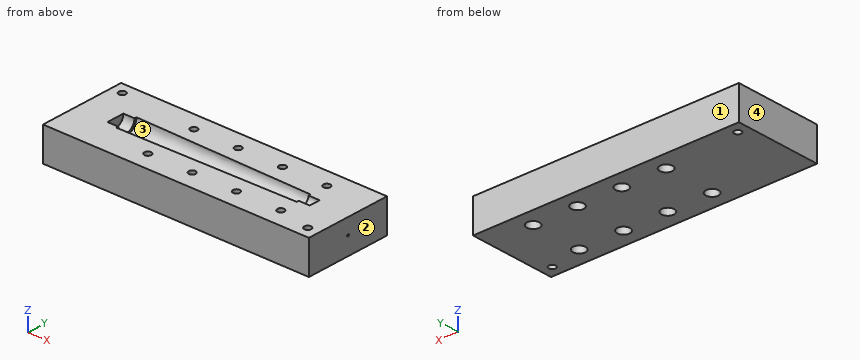
```python
from build123d import *

# Parameters (mm, degrees)
SKIZZE2_W                        = 120
SKIZZE2_H                        = 39.364160046
AUFSATZ_LINEAR_AUSTRAGEN1_DEPTH  = 30
SKIZZE24_R                       = 1.55
SCHNITT_LINEAR_AUSTRAGEN4_DEPTH  = 130.805766806
SKIZZE46_R                       = 2.85
SCHNITT_LINEAR_AUSTRAGEN15_DEPTH = 10
SCHNITT_LINEAR_START             = -5
SCHNITT_LINEAR_AUSTRAGEN25_DEPTH = 2.7
LINEARES_MUSTER1_COUNT           = 4
LINEARES_MUSTER1_PITCH           = 20
SPIEGELN2_COPY_1_SKETCH_R        = 2.85
SPIEGELN2_COPY_1_DEPTH           = 10
SPIEGELN2_COPY_2_SKETCH_R        = 2.85
SPIEGELN2_COPY_2_DEPTH           = 10
SPIEGELN2_COPY_3_SKETCH_R        = 2.85
SPIEGELN2_COPY_3_DEPTH           = 10
SPIEGELN2_START                  = -5
SPIEGELN2_COPY_4_DEPTH           = 2.7
SPIEGELN2_COPY_5_DEPTH           = 2.7
SPIEGELN2_COPY_6_DEPTH           = 2.7
SKIZZE51_R                       = 1.55
SCHNITT_LINEAR_AUSTRAGEN26_DEPTH = 130.805766806
SKIZZE75_R                       = 0.75
SCHNITT_LINEAR_AUSTRAGEN28_DEPTH = 10
SKIZZE76_R                       = 2
SCHNITT_LINEAR_AUSTRAGEN29_DEPTH = 6
SKIZZE80_R                       = 0.5
SCHNITT_LINEAR_AUSTRAGEN34_DEPTH = 21
SCHNITT_LINEAR_START_2           = -7.5
SKIZZE81_R                       = 0.5
SCHNITT_LINEAR_AUSTRAGEN36_DEPTH = 5
ABSPALTEN3_START                 = 15
ABSPALTEN3_OUTLINE_W             = 120
ABSPALTEN3_OUTLINE_H             = 39.364160046
ABSPALTEN3_OUTLINE_R             = 1.55
ABSPALTEN3_DEPTH                 = 15


# Read off the part's stored shape, not the designer's step: Abspalten3
with BuildPart() as part:
    # Skizze2 → Aufsatz-Linear austragen1 (new body)
    with BuildSketch(Plane.XY):
        with Locations((60, 19.682080023)):
            Rectangle(SKIZZE2_W, SKIZZE2_H)
    extrude(amount=AUFSATZ_LINEAR_AUSTRAGEN1_DEPTH)

    # Skizze24 → Schnitt-Linear austragen4 (cut, through all)
    with BuildSketch(Plane.XY.offset(30)):
        with Locations((40, 31.364160046)):
            Circle(SKIZZE24_R)
        with Locations((60, 31.364160046)):
            Circle(SKIZZE24_R)
        with Locations((80, 31.364160046)):
            Circle(SKIZZE24_R)
        with Locations((100, 31.364160046)):
            Circle(SKIZZE24_R)
    schnitt_linear_austragen4 = extrude(amount=-SCHNITT_LINEAR_AUSTRAGEN4_DEPTH, mode=Mode.SUBTRACT)

    # Skizze46 → Schnitt-Linear austragen15 (cut)
    with BuildSketch(Plane(origin=(0, 0, 0), x_dir=(-1, 0, 0), z_dir=(0, 0, -1))):
        with Locations((-100, 31.364160046)):
            Circle(SKIZZE46_R)
    schnitt_linear_austragen15 = extrude(amount=-SCHNITT_LINEAR_AUSTRAGEN15_DEPTH, mode=Mode.SUBTRACT)

    # Skizze50 → Schnitt-Linear austragen25 (cut)
    with BuildSketch(Plane.XY.offset(30).offset(SCHNITT_LINEAR_START)):
        Polygon((97.15, 33.009608314), (97.15, 39.364160046), (102.85, 39.364160046), (102.85, 33.009608314), (102.85, 29.718711779), (100, 28.073263512), (97.15, 29.718711779), align=None)
    schnitt_linear_austragen25 = extrude(amount=-SCHNITT_LINEAR_AUSTRAGEN25_DEPTH, mode=Mode.SUBTRACT)

    # Lineares Muster1: Schnitt-Linear austragen15, Schnitt-Linear austragen25 ×4
    with Locations(*[(-i * LINEARES_MUSTER1_PITCH, 0, 0) for i in range(1, LINEARES_MUSTER1_COUNT)]):
        add(schnitt_linear_austragen15, mode=Mode.SUBTRACT)
        add(schnitt_linear_austragen25, mode=Mode.SUBTRACT)

    # Spiegeln2: Schnitt-Linear austragen15, Schnitt-Linear austragen25 across plane
    add(schnitt_linear_austragen15.mirror(Plane.ZX.offset(19.764160046)), mode=Mode.SUBTRACT)
    add(schnitt_linear_austragen25.mirror(Plane.ZX.offset(19.764160046)), mode=Mode.SUBTRACT)

    # Spiegeln2 copy 1 sketch → Spiegeln2 copy 1 (cut)
    with BuildSketch(Plane(origin=(-20, 39.528320093, 0), x_dir=(-1, 0, 0), z_dir=(0, 0, -1))):
        with Locations((-100, -31.364160046)):
            Circle(SPIEGELN2_COPY_1_SKETCH_R)
    extrude(amount=-SPIEGELN2_COPY_1_DEPTH, mode=Mode.SUBTRACT)

    # Spiegeln2 copy 2 sketch → Spiegeln2 copy 2 (cut)
    with BuildSketch(Plane(origin=(-40, 39.528320093, 0), x_dir=(-1, 0, 0), z_dir=(0, 0, -1))):
        with Locations((-100, -31.364160046)):
            Circle(SPIEGELN2_COPY_2_SKETCH_R)
    extrude(amount=-SPIEGELN2_COPY_2_DEPTH, mode=Mode.SUBTRACT)

    # Spiegeln2 copy 3 sketch → Spiegeln2 copy 3 (cut)
    with BuildSketch(Plane(origin=(-60, 39.528320093, 0), x_dir=(-1, 0, 0), z_dir=(0, 0, -1))):
        with Locations((-100, -31.364160046)):
            Circle(SPIEGELN2_COPY_3_SKETCH_R)
    extrude(amount=-SPIEGELN2_COPY_3_DEPTH, mode=Mode.SUBTRACT)

    # Spiegeln2 copy 4 sketch → Spiegeln2 copy 4 (cut)
    with BuildSketch(Plane(origin=(-20, 39.528320093, 30), x_dir=(1, 0, 0), z_dir=(0, 0, 1)).offset(SPIEGELN2_START)):
        Polygon((97.15, -33.009608314), (97.15, -39.364160046), (102.85, -39.364160046), (102.85, -33.009608314), (102.85, -29.718711779), (100, -28.073263512), (97.15, -29.718711779), align=None)
    extrude(amount=-SPIEGELN2_COPY_4_DEPTH, mode=Mode.SUBTRACT)

    # Spiegeln2 copy 5 sketch → Spiegeln2 copy 5 (cut)
    with BuildSketch(Plane(origin=(-40, 39.528320093, 30), x_dir=(1, 0, 0), z_dir=(0, 0, 1)).offset(SPIEGELN2_START)):
        Polygon((97.15, -33.009608314), (97.15, -39.364160046), (102.85, -39.364160046), (102.85, -33.009608314), (102.85, -29.718711779), (100, -28.073263512), (97.15, -29.718711779), align=None)
    extrude(amount=-SPIEGELN2_COPY_5_DEPTH, mode=Mode.SUBTRACT)

    # Spiegeln2 copy 6 sketch → Spiegeln2 copy 6 (cut)
    with BuildSketch(Plane(origin=(-60, 39.528320093, 30), x_dir=(1, 0, 0), z_dir=(0, 0, 1)).offset(SPIEGELN2_START)):
        Polygon((97.15, -33.009608314), (97.15, -39.364160046), (102.85, -39.364160046), (102.85, -33.009608314), (102.85, -29.718711779), (100, -28.073263512), (97.15, -29.718711779), align=None)
    extrude(amount=-SPIEGELN2_COPY_6_DEPTH, mode=Mode.SUBTRACT)

    # Spiegeln3: Schnitt-Linear austragen4 across plane
    add(schnitt_linear_austragen4.mirror(Plane.ZX.offset(19.764160046)), mode=Mode.SUBTRACT)

    # Skizze51 → Schnitt-Linear austragen26 (cut, through all)
    with BuildSketch(Plane.XY.offset(30)):
        with Locations((5, 34.364160046)):
            Circle(SKIZZE51_R)
        with Locations((115, 5)):
            Circle(SKIZZE51_R)
    extrude(amount=-SCHNITT_LINEAR_AUSTRAGEN26_DEPTH, mode=Mode.SUBTRACT)

    # Skizze73 → Schnitt-Rotation5 (revolve, cut)
    with BuildSketch(Plane.XY.offset(15)):
        Polygon((15, 19.764160046), (15, 23.764160046), (20, 23.764160046), (20, 24.764160046), (100, 23.182080023), (100, 22.182080023), (105, 22.182080023), (105, 19.682080023), align=None)
    revolve(axis=Axis((105, 19.682080023, 15), (-0.9999995841280241, 0.0009119998787298228, 0)), mode=Mode.SUBTRACT)

    # Skizze75 → Schnitt-Linear austragen28 (cut)
    with BuildSketch(Plane.XY.offset(30)):
        with Locations((21.598259807, 19.682080023)):
            Circle(SKIZZE75_R)
    extrude(amount=-SCHNITT_LINEAR_AUSTRAGEN28_DEPTH, mode=Mode.SUBTRACT)

    # Skizze76 → Schnitt-Linear austragen29 (cut)
    with BuildSketch(Plane.XY.offset(30)):
        with Locations((21.598259807, 19.682080023)):
            Circle(SKIZZE76_R)
    extrude(amount=-SCHNITT_LINEAR_AUSTRAGEN29_DEPTH, mode=Mode.SUBTRACT)

    # Skizze80 → Schnitt-Linear austragen34 (cut)
    with BuildSketch(Plane(origin=(120, 0, 0), x_dir=(0, 0, -1), z_dir=(1, 0, 0))):
        with Locations((-22.000416524, 19.763714623)):
            Circle(SKIZZE80_R)
    schnitt_linear_austragen34 = extrude(amount=-SCHNITT_LINEAR_AUSTRAGEN34_DEPTH, mode=Mode.SUBTRACT)

    # Skizze81 → Schnitt-Linear austragen36 (cut)
    with BuildSketch(Plane.XY.offset(30).offset(SCHNITT_LINEAR_START_2)):
        with Locations(Location((99, 19.682080023, 0), (0, 0, 7.034090001))):
            Circle(SKIZZE81_R)
    schnitt_linear_austragen36 = extrude(amount=-SCHNITT_LINEAR_AUSTRAGEN36_DEPTH, mode=Mode.SUBTRACT)

    # Spiegeln4: Schnitt-Linear austragen34, Schnitt-Linear austragen36 across plane
    add(schnitt_linear_austragen34.mirror(Plane.XY.offset(15)), mode=Mode.SUBTRACT)
    add(schnitt_linear_austragen36.mirror(Plane.XY.offset(15)), mode=Mode.SUBTRACT)

    # Abspalten3 outline → Abspalten3 (cut)
    with BuildSketch(Plane.XY.offset(ABSPALTEN3_START)):
        with Locations((60, 19.682080023)):
            Rectangle(ABSPALTEN3_OUTLINE_W, ABSPALTEN3_OUTLINE_H)
        with Locations((115, 5)):
            Circle(ABSPALTEN3_OUTLINE_R, mode=Mode.SUBTRACT)
        with Locations((5, 34.364160046)):
            Circle(ABSPALTEN3_OUTLINE_R, mode=Mode.SUBTRACT)
        with Locations((40, 31.364160046)):
            Circle(ABSPALTEN3_OUTLINE_R, mode=Mode.SUBTRACT)
        with Locations((60, 31.364160046)):
            Circle(ABSPALTEN3_OUTLINE_R, mode=Mode.SUBTRACT)
        with Locations((80, 31.364160046)):
            Circle(ABSPALTEN3_OUTLINE_R, mode=Mode.SUBTRACT)
        with Locations((100, 31.364160046)):
            Circle(ABSPALTEN3_OUTLINE_R, mode=Mode.SUBTRACT)
        with Locations((40, 8.164160046)):
            Circle(ABSPALTEN3_OUTLINE_R, mode=Mode.SUBTRACT)
        with Locations((60, 8.164160046)):
            Circle(ABSPALTEN3_OUTLINE_R, mode=Mode.SUBTRACT)
        with Locations((80, 8.164160046)):
            Circle(ABSPALTEN3_OUTLINE_R, mode=Mode.SUBTRACT)
        with Locations((100, 8.164160046)):
            Circle(ABSPALTEN3_OUTLINE_R, mode=Mode.SUBTRACT)
    extrude(amount=ABSPALTEN3_DEPTH, mode=Mode.SUBTRACT)


solid = part.part
```
Input: part model. Units: mm. Frame: model coordinates. Face numbers are marked on the shaded views. Round coordinates to 2 decimals unless told otherwise and drop trailing zeros. Loops run counter-clockwise (first coordinate to the right, second up) from the corner with the lowest first, then second, coordinate; pieces in that order, holes last. Notation, with made-up numbers: (-39, 12.5) -> (0, 12.5) arc R25 ccw to (0, 41.5) -> close; hole circle Ø2 at (48.5, 28). An arc over 180 degrees is marked (long way). Use one line per item in the form item = value. Start each with the question number.
Item 1: Section query C-C on z = 4. Count the separate pieces of the cut face and the enclosed holes in it, then the cut area to 3 significant figures.
Item 2: Contact query for flat-ended pins moving along their axis: pin 1 Ø1.7 at (x, y) = (101.5, 7) entering from -Z; pin 2 Ø1 at (x, y) = (24, 19) entering from +Z. Output: stop coordinate, or through.
Item 3: Section query A-A on x = 115. Return the cut outline in (y, z).
Item 4: Mould query, pull axis X, two halves, no side actions, for the marked faces 1, 2, 3 and 4. Classes: pulls with the +X half, pulls with the -X half, needs draft (parallel to the pull), parting line crosses it, or undercut.
Item 5: Material intervals for L1, parallel to Y at x = 40, z = 7.5; L2, parallel to X at y = 8.5, z = 3; L3, parallel to X at y = 9.5, z = 4, sorted ascending. Write a range as from..to.
Item 6: Section query B-B on x = 5. Return the cut outline in (y, z), then the cut area to 3 significant figures.
Ans:
q1.separate_pieces = 1
q1.enclosed_holes = 10
q1.area = 4,500 mm^2
q2.pin_1 = 10
q2.pin_2 = 10.23
q3.outline = (0, 0) -> (3.45, 0) -> (3.45, 15) -> (0, 15) -> close; (6.55, 0) -> (39.36, 0) -> (39.36, 15) -> (6.55, 15) -> close; hole circle Ø1 at (19.76, 8)
q4.face_1 = needs draft
q4.face_2 = pulls with the +X half
q4.face_3 = undercut
q4.face_4 = pulls with the -X half
q5.L1 = 0..5.31, 11.01..28.51, 34.21..39.36
q5.L2 = 0..37.17, 42.83..57.17, 62.83..77.17, 82.83..97.17, 102.83..120
q5.L3 = 0..37.48, 42.52..57.48, 62.52..77.48, 82.52..97.48, 102.52..120
q6.outline = (0, 0) -> (32.81, 0) -> (32.81, 15) -> (0, 15) -> close; (35.91, 0) -> (39.36, 0) -> (39.36, 15) -> (35.91, 15) -> close
q6.area = 544 mm^2
